The model under review builds one solid part; all positions refer to its coordinate system, in mm. A direction names the side the tool comes from. Round coordinates to 2 decimals unless told otherwise and drop trailing zeros. Write each loop counter-clockwise with the first axis right and the second up, starting at its lowest first coordinate (ties: lowest second). Pieces come first, ordered by that corner, then holes. Notation, with made-up numbers: (-6, -5) - (30, -5) arc R30 cw to (30, 23) - close; hole circle Ø1 at (-30.5, -39). An arc over 180 degrees is marked (long way). Return JSON: item names as keys, results as strings.
from build123d import *

# Parameters (mm, degrees)
SKETCH1_R           = 8
BOSS_EXTRUDE2_DEPTH = 37
SKETCH4_R           = 10.5
BOSS_EXTRUDE4_DEPTH = 50
SHELL1_T            = -1
CUT_EXTRUDE2_REACH  = 90.258
SKETCH5_R           = 9.5


with BuildPart() as part:
    # Sketch1 → Boss-Extrude2 (new body)
    with BuildSketch(Plane.XY):
        Circle(SKETCH1_R)
    extrude(amount=BOSS_EXTRUDE2_DEPTH)

    # Sketch4 → Boss-Extrude4 (add)
    with BuildSketch(Plane(origin=(0, 0, 0), x_dir=(-1, 0, 0), z_dir=(0, 0, -1))):
        Circle(SKETCH4_R)
    extrude(amount=BOSS_EXTRUDE4_DEPTH)

    # Shell1
    shell1_openings = [part.faces().sort_by_distance(p)[0] for p in [
        (0, 0, 37),
    ]]
    offset(amount=SHELL1_T, openings=shell1_openings, kind=Kind.INTERSECTION)

    # Sketch5 → Cut-Extrude2 (cut, up to next)
    with BuildSketch(Plane(origin=(0, 0, -50), x_dir=(-1, 0, 0), z_dir=(0, 0, -1)), mode=Mode.PRIVATE) as cut_extrude2_sk1:
        Circle(SKETCH5_R)
    cut_extrude2_tool1 = extrude(cut_extrude2_sk1.sketch, amount=-CUT_EXTRUDE2_REACH, mode=Mode.PRIVATE) & part.part
    add(cut_extrude2_tool1.solids().sort_by_distance((0, 0, -50))[0], mode=Mode.SUBTRACT)


solid = part.part
(1) Mouldability with a two-part tool opening along X and no side actions: class faces 1 (the flat face through (4, -6, -1)), 2 (the cylindrical face through (-10, 3.2, -24.6)), 3 (the flat face through (2, -8, 0)) as released by +X, released by -X, zero draft, split by the parting line, or undercut.
Filled in:
{"face 1": "undercut", "face 2": "split by the parting line", "face 3": "zero draft"}
(2) Wall thickness on line 1 (Y direction, x = 0, z = 8.5); line 2 (Y direction, x = 0, z = -21); line 3 (X direction, y = 2.5, z = -46): over which ranges is each line inside the solid? List them lowest first.
Filled in:
{"line 1": "y = -8 to -7, 7 to 8", "line 2": "y = -10.5 to -9.5, 9.5 to 10.5", "line 3": "x = -10.2 to -9.17, 9.17 to 10.2"}
(3) For faces 4 (the flat face through (5, -9, -50)), 5 (the cylindrical face through (-1.73, -7.81, 18.24)), 6 (the cylindrical face through (-4.38, -8.43, -25.84)), list the 3-axis set-ups (+Z, -Z, +X, -X, +Y, -Y) from which the entire face can be reached by the end or side of a thin tool; tool diameter is ignored.
Filled in:
{"face 4": "-Z, +X, -X, +Y, -Y", "face 5": "+Z", "face 6": "-Z"}
(4) Clearance check with flat-ended pins moving along their axes: pin 1 Ø12 at (x, z) = (-7, 18.5) entering from -Y; pin 2 Ø2 at (y, z) = (4, 22) entering from +X; pin 3 Ø10 at (x, z) = (7.5, -1) entering from +Y; pin 4 Ø12.5 at (x, y) = (0, 0) entering from +Z. State where each tip first meets the part, or that it passes through.
Filled in:
{"pin 1": "stops at y = -7.94", "pin 2": "stops at x = 7.42", "pin 3": "stops at y = 10.2", "pin 4": "passes through"}
(5) Add section A-A (y = 0). Write out the cut boundary in (x, z).
Filled in:
{"outline": "(-10.5, -50) - (-9.5, -50) - (-9.5, -1) - (-7, -1) - (-7, 37) - (-8, 37) - (-8, 0) - (-10.5, 0) - close; (7, -1) - (9.5, -1) - (9.5, -50) - (10.5, -50) - (10.5, 0) - (8, 0) - (8, 37) - (7, 37) - close"}
(6) Add section D-D (z = -45). Write out the cut boundary in (x, y).
Filled in:
{"outline": "circle Ø21 at (0, 0); hole circle Ø19 at (0, 0)"}
(7) Add section C-C (z = 5). Write out the cut boundary in (x, y).
Filled in:
{"outline": "circle Ø16 at (0, 0); hole circle Ø14 at (0, 0)"}
